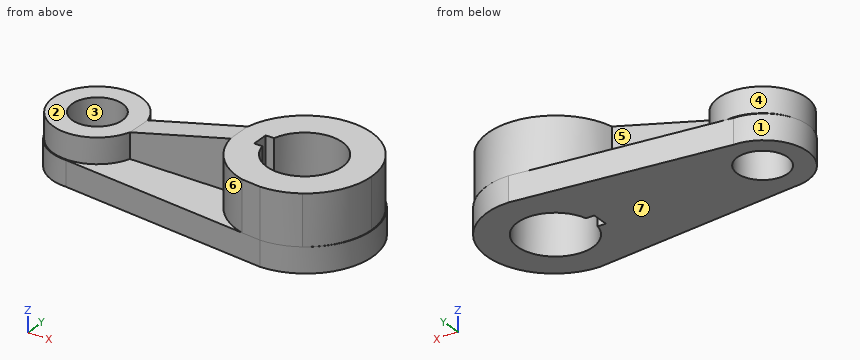
from build123d import *

# Parameters (mm, degrees)
BOSS_EXTRUDE1_DEPTH     = 12
SKETCH7_R               = 21
BOSS_EXTRUDE3_DEPTH     = 12
BOSS_EXTRUDE4_START     = 24
BOSS_EXTRUDE4_DEPTH     = 24
SKETCH9_R               = 12
SKETCH9_R_2             = 18
CUT_EXTRUDE1_DEPTH      = 94.856036825
CUT_EXTRUDE2_DEPTH      = 94.856036825
CUT_EXTRUDE2_DEPTH_BACK = 94.856036825
SKETCH9_3_R             = 12
SKETCH9_3_R_2           = 18
CUT_EXTRUDE3_DEPTH      = 98.616369777
CUT_EXTRUDE3_DEPTH_BACK = 98.616369777
BOSS_EXTRUDE5_DEPTH     = 24
CUT_EXTRUDE4_DEPTH      = 97.067453638
CUT_EXTRUDE4_DEPTH_BACK = 24


with BuildPart() as part:
    # Sketch4 → Boss-Extrude1 (new body)
    with BuildSketch(Plane.XY):
        with BuildLine():
            ThreePointArc((-47.094430993, 21), (-68.094430993, 0), (-47.094430993, -21))
            Line((-47.094430993, -21), (52.905569007, -32))
            ThreePointArc((52.905569007, -32), (84.905569007, 0), (52.905569007, 32))
            Line((52.905569007, 32), (-47.094430993, 21))
        make_face()
    extrude(amount=-BOSS_EXTRUDE1_DEPTH)

    # Sketch7 → Boss-Extrude3 (add)
    with BuildSketch(Plane.XY):
        with Locations(Location((-46.916866089, 0.498400316, 0), (0, 0, 161.112350505))):
            Circle(SKETCH7_R)
    extrude(amount=BOSS_EXTRUDE3_DEPTH)

    # Sketch7_4 → Boss-Extrude4 (add)
    with BuildSketch(Plane.XY.offset(BOSS_EXTRUDE4_START)):
        with BuildLine():
            ThreePointArc((69.890228484, -27.120496722), (80.621286149, -15.545614643), (84.513996989, -0.249200158))
            ThreePointArc((84.513996989, -0.249200158), (33.309113789, 25.347136714), (43.56571816, -30.972616407))
            Line((43.56571816, -30.972616407), (52.905569007, -32))
            ThreePointArc((52.905569007, -32), (61.741408099, -30.755941663), (69.890228484, -27.120496722))
        make_face()
    extrude(amount=-BOSS_EXTRUDE4_DEPTH)

    # Sketch9 → Cut-Extrude1 (cut, through all)
    with BuildSketch(Plane.XY):
        with Locations((-46.916866089, 0.498400316)):
            Circle(SKETCH9_R)
        with Locations((52.513996989, -0.249200158)):
            Circle(SKETCH9_R_2)
    extrude(amount=-CUT_EXTRUDE1_DEPTH, mode=Mode.SUBTRACT)

    # Sketch9_3 → Cut-Extrude2 (cut, two sides: drawn at the far end of the back side and taken through both)
    with BuildSketch(Plane.XY.offset(-CUT_EXTRUDE2_DEPTH_BACK)):
        with Locations((-46.916866089, 0.498400316)):
            Circle(SKETCH9_3_R)
        with Locations((52.513996989, -0.249200158)):
            Circle(SKETCH9_3_R_2)
    extrude(amount=CUT_EXTRUDE2_DEPTH + CUT_EXTRUDE2_DEPTH_BACK, mode=Mode.SUBTRACT)

    # Sketch10 → Cut-Extrude3 (cut, two sides: drawn at the far end of the back side and taken through both)
    with BuildSketch(Plane.XY.offset(24).offset(-CUT_EXTRUDE3_DEPTH_BACK)):
        Polygon((35.022733512, 4), (31.022733512, 4), (31.022733512, -4), (34.909125489, -4), align=None)
    extrude(amount=CUT_EXTRUDE3_DEPTH + CUT_EXTRUDE3_DEPTH_BACK, mode=Mode.SUBTRACT)

    # Sketch11 → Boss-Extrude5 (add)
    with BuildSketch(Plane.XY):
        Polygon((-26.650332075, 6), (21.130123784, 6), (21.034983326, -6), (-26.9476199, -6), align=None)
    extrude(amount=BOSS_EXTRUDE5_DEPTH)

    # Sketch12 → Cut-Extrude4 (cut, two sides: drawn at the far end of the back side and taken through both)
    with BuildSketch(Plane.XZ.offset(6).offset(-CUT_EXTRUDE4_DEPTH_BACK)):
        Polygon((21.034983326, 24), (-26.9476199, 12), (-26.9476199, 24), align=None)
    extrude(amount=CUT_EXTRUDE4_DEPTH + CUT_EXTRUDE4_DEPTH_BACK, mode=Mode.SUBTRACT)


solid = part.part
For this review, take the finished solid that the model builds, in its own axes (mm). Face numbers are marked on the shaded views. A direction names the side the tool comes from. Round coordinates to 2 decimals unless told otherwise and drop trailing zeros. Loops run counter-clockwise (first coordinate to the right, second up) from the corner with the lowest first, then second, coordinate; pieces in that order, holes last. Notation, with made-up numbers: (66, 89.5) - (108, 89.5) arc R15 ccw to (108, 109.5) - close; hole circle Ø5 at (42.25, 5). An arc over 180 degrees is marked (long way). One line per item, written item: value. Start each with the question number.
Item 1: Take a section at B-B (y = 27.5). Give the boundary of the cut face in (x, z).
Item 2: Clearance check with flat-ended pins moving along their axes: pin 1 Ø12 at (y, z) = (-11.5, 3) entering from +X; pin 2 Ø4 at (x, y) = (-11, -10) entering from +Z; pin 3 Ø5 at (x, z) = (-2.5, -1.5) entering from -Y; pin 4 Ø12 at (x, y) = (25, -17) entering from +Z. State where each tip first meets the part, or that it passes through.
Item 3: Take a section at A-A (z = 2.5). Give the boundary of the cut face in (x, y), plus the area to 3 significant figures.
Item 4: Take a section at C-C (x = -12.5). Give the boundary of the cut face in (y, z).
Item 5: For the marked faces 4, 5, 6 and 7, list the 3-axis set-ups (+Z, -Z, +X, -X, +Y, -Y) from which the entire face can be reached by the end or side of a thin tool; tool diameter is ignored.
Item 6: The part is to be moulded in two halves that separate along X. For the marked faces 1, 2 and 3, say which applies: +X half, -X half, draft (parallel to the pull), parting line (faces both ways), or undercut.
Item 7: For L1, parallel to X at y = 0, z = -9.5; L2, parallel to X at y = -14.5, z = 6.5; L3, parallel to X at y = 10, z = 0.5, list the stretches that pass through material, from the lowest coordinate up.
Item 8: Take a section at D-D (z = -4). Give the boundary of the cut face in (x, y), plus the area to 3 significant figures.
Answer below:
1. outline: (12, -12) - (69.27, -12) - (69.27, 0) - (68.45, 0) - (68.45, 24) - (36.58, 24) - (36.58, 0) - (12, 0) - close
2. pin 1: stops at x = 84.28
2. pin 2: stops at z = 0
2. pin 3: stops at y = -26.18
2. pin 4: stops at z = 24
3. outline: (-26.95, -6) - (21.03, -6) arc R32 ccw to (43.57, -30.97) - (52.91, -32) arc R32 ccw to (69.89, -27.12) arc R32 ccw (long way) to (21.13, 6) - (-26.65, 6) arc R21 ccw (long way) to start; hole circle Ø24 at (-46.92, 0.5); hole (31.02, -4) - (34.91, -4) arc R18 ccw (long way) to (35.02, 4) - (31.02, 4) - close
3. area: 3,660 mm2
4. outline: (-24.81, -12) - (24.81, -12) - (24.81, 0) - (6, 0) - (6, 15.61) - (-6, 15.61) - (-6, 0) - (-24.81, 0) - close
5. face 4: +Z
5. face 5: +Z, +Y
5. face 6: +Z, -Y
5. face 7: -Z, +X, -X, +Y, -Y
6. face 1: -X half
6. face 2: draft
6. face 3: undercut
7. L1: x = -68.09 to -58.91, -34.93 to 31.02, 70.51 to 84.91
7. L2: x = -61.62 to -32.22, 23.86 to 41.52, 63.51 to 81.17
7. L3: x = -65.64 to -54.25, -39.59 to -28.19, 22.2 to 37.72, 67.31 to 82.83
8. outline: (-47.09, -21) - (52.91, -32) arc R32 ccw to (52.91, 32) - (-47.09, 21) arc R21 ccw to start; hole circle Ø24 at (-46.92, 0.5); hole (31.02, -4) - (34.91, -4) arc R18 ccw (long way) to (35.02, 4) - (31.02, 4) - close
8. area: 6,100 mm2
